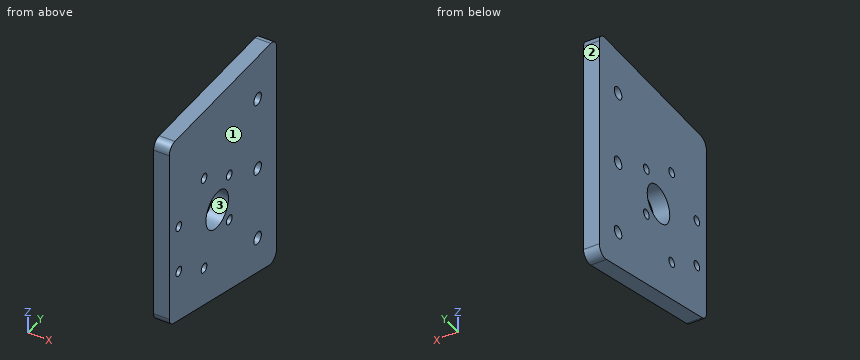
from build123d import *

# Parameters (mm, degrees)
SKETCH1_R           = 6
SKETCH1_R_2         = 2
SKETCH1_R_3         = 1.5
BOSS_EXTRUDE1_DEPTH = 5
FILLET1_R           = 3


with BuildPart() as part:
    # Sketch1 → Boss-Extrude1 (new body)
    with BuildSketch(Plane(origin=(0, 0, 0), x_dir=(0, 0, -1), z_dir=(1, 0, 0))):
        Polygon((0, 0), (77, 0), (61.726896031, -57), (0, -57), align=None)
        with Locations((38.5, -31.5)):
            Circle(SKETCH1_R, mode=Mode.SUBTRACT)
        with Locations((38.5, -10)):
            Circle(SKETCH1_R_2, mode=Mode.SUBTRACT)
        with Locations((62.5, -10)):
            Circle(SKETCH1_R_2, mode=Mode.SUBTRACT)
        with Locations((14.5, -10)):
            Circle(SKETCH1_R_2, mode=Mode.SUBTRACT)
        with Locations((23, -38.5)):
            Circle(SKETCH1_R_3, mode=Mode.SUBTRACT)
        with Locations((30.75, -25.076606241)):
            Circle(SKETCH1_R_3, mode=Mode.SUBTRACT)
        with Locations((46.25, -25.076606241)):
            Circle(SKETCH1_R_3, mode=Mode.SUBTRACT)
        with Locations((54, -38.5)):
            Circle(SKETCH1_R_3, mode=Mode.SUBTRACT)
        with Locations((46.25, -51.923393759)):
            Circle(SKETCH1_R_3, mode=Mode.SUBTRACT)
        with Locations((30.75, -51.923393759)):
            Circle(SKETCH1_R_3, mode=Mode.SUBTRACT)
    extrude(amount=BOSS_EXTRUDE1_DEPTH)

    # Fillet1
    fillet1_edges = [part.edges().sort_by_distance(p)[0] for p in [
        (2.5, 0, 0),
        (2.5, 0, -77),
        (2.5, -57, -61.726896031),
        (2.5, -57, 0),
    ]]
    fillet(fillet1_edges, radius=FILLET1_R)


solid = part.part
Verification items for the finished model (mm, model axes). Face numbers are marked on the shaded views. Give positions to 0.01 mm unless a question says otherwise; leave off trailing zeros. Order: outer loops, then holes, each group sorted by start corner. A loop starts at its lowest first (then second) coordinate and runs counter-clockwise, first axis right, second up. Notation, with made-up numbers: M 82,41.5 L 141,41.5 A26 ccw 141,67.5 Z; hole C -14.5,17 d9. An arc over 180 degrees is marked long. Use one line per item in the form item = value. Start each with the question number.
Q1. Section check C-C (z = -46.25). Enter the section's corners in (x, y).
Q2. Scan lines: line 1 along Y through (x, z) = (1.1, -30.75); line 2 along Z through (x, y) = (0.55, -51.5); line 3 along Y through (x, z) = (3.25, -45). Record each from-to range of solid material in increasing order. Write a range as [from, to].
Q3. Section check D-D (y = -31.5). Enter the section's corners in (x, z).
Q4. Section check B-B (y = -38.5). Enter the section's corners in (x, z).
Q5. Mould release check, pull along Y, two halves, no side actions. Record for the marked faces 1, 2 and 3: +Y half, -Y half, draft (parallel to the pull), parting line (faces both ways), or undercut.
Q6. Section check A-A (z = -23). Enter the section's corners in (x, y), then the cut area to 3 significant figures.
Evaluation:
q1.outline = M 0,-57 L 5,-57 L 5,-53.42 L 0,-53.42 Z; M 0,-50.42 L 5,-50.42 L 5,-26.58 L 0,-26.58 Z; M 0,-23.58 L 5,-23.58 L 5,0 L 0,0 Z
q2.line_1 = [-57, -53.42], [-50.42, -26.58], [-23.58, 0]
q2.line_2 = [-63.2, -47.69], [-44.81, -32.19], [-29.31, 0]
q2.line_3 = [-57, -52.75], [-51.09, -25.91], [-24.25, 0]
q3.outline = M 0,-68.56 L 5,-68.56 L 5,-44.5 L 0,-44.5 Z; M 0,-32.5 L 5,-32.5 L 5,0 L 0,0 Z
q4.outline = M 0,-66.68 L 5,-66.68 L 5,-55.5 L 0,-55.5 Z; M 0,-52.5 L 5,-52.5 L 5,-24.5 L 0,-24.5 Z; M 0,-21.5 L 5,-21.5 L 5,0 L 0,0 Z
q5.face_1 = draft
q5.face_2 = +Y half
q5.face_3 = undercut
q6.outline = M 0,-57 L 5,-57 L 5,-40 L 0,-40 Z; M 0,-37 L 5,-37 L 5,0 L 0,0 Z
q6.area = 270 mm2
